Autodesk Inventor part; units mm, degrees
ref_plane "YZ Plane" through (0, 0, 0) normal (1, 0, 0) x (0, 1, 0)
ref_plane "XZ Plane" through (0, 0, 0) normal (0, 1, 0) x (-1, 0, 0)
ref_plane "XY Plane" through (0, 0, 0) normal (0, 0, 1) x (1, 0, 0)
sketch "Master_XZ" plane through (0, 0, 0) normal (0, 1, 0) x (-1, 0, 0)
  line L0 (52.5, 47.5) -> (-52.5, 47.5)
  line L1 (-52.5, 47.5) -> (-52.5, -47.5)
  line L2 (-52.5, -47.5) -> (52.5, -47.5)
  line L3 (52.5, -47.5) -> (52.5, 47.5)
  line L4 (52.5, 47.5) -> (-52.5, -47.5) construction
  line L5 (-52.5, 47.5) -> (52.5, -47.5) construction
  line L6 (50.5, 45.5) -> (-50.5, 45.5)
  line L7 (-50.5, 45.5) -> (-50.5, -45.5)
  line L8 (-50.5, -45.5) -> (50.5, -45.5)
  line L9 (50.5, -45.5) -> (50.5, 45.5)
  line L10 (48.5, 43.5) -> (-48.5, 43.5)
  line L11 (-48.5, 43.5) -> (-48.5, -43.5)
  line L12 (-48.5, -43.5) -> (48.5, -43.5)
  line L13 (48.5, -43.5) -> (48.5, 43.5)
  point P0 (0, 0)
  dimension "d0" = 2
  dimension "d1" = 2
  dimension "d10" = 105
  dimension "d15" = 95
extrude "Floor" add sketch "Master_XZ" along normal blind 2 contours L3 L2 L1 L0 | L9 L8 L7 L6 | L13 L12 L11 L10
extrude "Walls" add sketch "Master_XZ" along normal blind 6 contours L9 L8 L7 L6
sketch "Lip_profile" plane through (0, 1, -41.5) normal (1, 0, 0) x (0, 0, -1)
  line L0 (-87, 1) -> (-87, 5)
  circle A0 centre (-87, 4) radius 1
  line L1 (-87, 5) -> (4, 5)
  line L2 (-87, 5) -> (-87, 3)
  point P0 (-41.5, -1)
  dimension "d6" = 2
  dimension "d7" = 1
extrude "Lip" add sketch "Lip_profile" along normal mid plane 100
sketch "Sketch3" plane through (50, 1, -41.5) normal (1, 0, 0) x (0, 0, -1)
  line L0 (-87, 5) -> (-87, 3)
  line L1 (-87, 5) -> (-87, 3)
  arc A0 (-87, 5) -> (-87, 3) centre (-87, 4) ccw
  point P0 (-41.5, -1)
revolve "Lip_edge_right" add sketch "Sketch3" angle 90 about axis through (50, 6, 45.5) along (0, 1, 0)
sketch "Sketch4" plane through (-50, 1, -41.5) normal (-1, 0, 0) x (0, 0, 1)
  line L0 (87, 3) -> (87, 5)
  arc A0 (87, 3) -> (87, 5) centre (87, 4) ccw
  point P0 (41.5, -1)
revolve "Lip_edge_left" add sketch "Sketch4" angle 90 about axis through (-50, 4, 45.5) along (0, -1, 0)
pattern_circular "Circular Pattern1" count 2 over 360 about axis through (0, -10, 0) along (0, 1, 0) of "Lip", "Lip_edge_right", "Lip_edge_left"
properties part number "BARB_bottom" material "ABS Plastic"
Work out the finished part from the listing and answer in its coordinate system (mm). A direction names the side the tool comes from. Give positions to 0.01 mm unless a question says otherwise; leave off trailing zeros. Write each loop counter-clockwise with the first axis right and the second up, starting at its lowest first coordinate (ties: lowest second). Pieces come first, ordered by that corner, then holes.
Q1. Given pin 1 (0.6 mm diameter, centred on x = -2.5, y = 3, fed in from +Z); pin 2 (1.2 mm diameter, centred on x = -5.5, y = 5, fed in from +Z); pin 3 (0.6 mm diameter, centred on x = 51, y = 4.5, fed in from -Z), each flat-ended and moving along its own axis, determine where each tip first touches the part or whether it passes through.
Answer:
pin 1: stops at z = 45.5
pin 2: stops at z = 46.5
pin 3: stops at z = -46.08
Q2. A tool of negligible diameter and unlimited length cuts with its end or side. For faces 1 (the face through (1, 2, 1)), 2 (the face through (-1, 3, 45.5)), 3 (the face through (50.5, 4, 1)), from which of +Z, -Z, +X, -X, +Y, -Y can it reach the whole face along a straight path? Write none if from no direction.
Answer:
face 1: +Y
face 2: +Z, +X, -X
face 3: +X, +Y
Q3. The part is cut by section B-B on z = -3. Give the vertices of the cut face in (x, y).
Answer:
outline: (-52.5, 0) - (52.5, 0) - (52.5, 2) - (50.5, 2) - (50.5, 6) - (48.5, 6) - (48.5, 2) - (-48.5, 2) - (-48.5, 6) - (-50.5, 6) - (-50.5, 2) - (-52.5, 2) - close
Q4. The part is cut by section C-C on x = -1. Give the vertices of the cut face in (y, z).
Answer:
outline: (0, -47.5) - (2, -47.5) - (2, -45.5) - (4, -45.5) arc R1 ccw to (6, -45.5) - (6, -43.5) - (2, -43.5) - (2, 43.5) - (6, 43.5) - (6, 45.5) arc R1 ccw to (4, 45.5) - (2, 45.5) - (2, 47.5) - (0, 47.5) - close
Q5. The part is cut by section A-A on y = 3.1. Give the vertices of the cut face in (x, z).
Answer:
outline: (-50.5, -45.5) - (50.5, -45.5) - (50.5, 45.5) - (-50.5, 45.5) - close; hole (-48.5, -43.5) - (48.5, -43.5) - (48.5, 43.5) - (-48.5, 43.5) - close
Q6. For a pull along Z with two mould halves and no side action, classify faces 4 (the face through (1, 3, -45.5)), 5 (the face through (51, 2, 0)), 6 (the face through (-50.5, 4, -1)) as released by +Z, released by -Z, zero draft, split by the parting line, or undercut.
Answer:
face 4: released by -Z
face 5: zero draft
face 6: undercut
Q7. Straight lines are drawn through the part: L1, parallel to X at y = 2.4, z = -18; L2, parallel to Z at x = -43, y = 5.2; L3, parallel to Z at x = 20, y = 3.85. For each, find the intervals that lie inside material, in ascending order.
Answer:
L1: x = -50.5 to -48.5, 48.5 to 50.5
L2: z = -46.48 to -43.5, 43.5 to 46.48
L3: z = -45.5 to -43.5, 43.5 to 45.5
